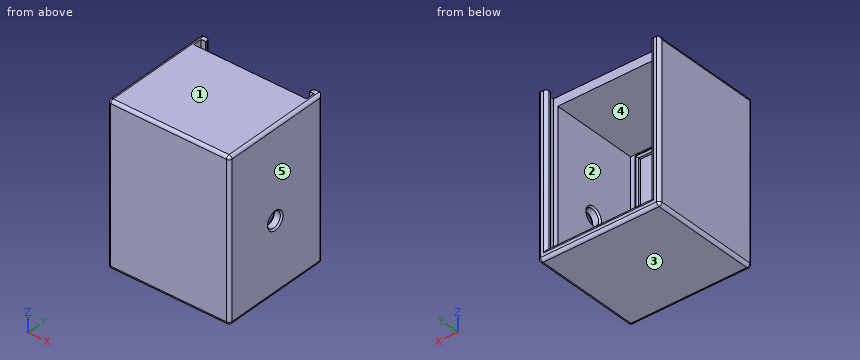
Autodesk Inventor part; units mm, degrees
ref_plane "Work Plane1" through (0, 0, 0) normal (0, 0, 1) x (1, 0, 0)
ref_plane "Work Plane2" through (0, 0, 0) normal (1, 0, 0) x (0, 1, 0)
ref_plane "XZ Plane" through (0, 0, 0) normal (0, 1, 0) x (-1, 0, 0)
sketch "Sketch1" plane through (0, 0, 0) normal (0, 0, 1) x (1, 0, 0)
  line L0 (-41, 37.5) -> (41, 37.5)
  line L1 (41, 37.5) -> (41, -37.5)
  line L2 (41, -37.5) -> (-41, -37.5)
  line L3 (-41, -37.5) -> (-41, 37.5)
  point P0 (0, 0)
  point P1 (0, 37.5)
  point P2 (-41, 0)
  dimension "d0" = 82
  dimension "d1" = 75
extrude "Extrusion1" add sketch "Sketch1" along normal mid plane 107
sketch "Sketch2" plane through (-41, 37.5, 53.5) normal (0, 1, 0) x (1, 0, 0)
  line L0 (0, 107) -> (82, 107)
  line L1 (6, 101) -> (76, 101)
  line L2 (76, 101) -> (76, 6)
  line L3 (76, 6) -> (6, 6)
  line L4 (6, 6) -> (6, 101)
  line L5 (0, 107) -> (0, 0)
  point P0 (41, 53.5)
  point P1 (41, 101)
  point P2 (41, 107)
  point P3 (6, 53.5)
  point P4 (0, 53.5)
  dimension "d4" = 95
  dimension "d5" = 70
extrude "Extrusion2" cut sketch "Sketch2" against normal blind 68
sketch "Sketch3" plane through (0, 0, 53.5) normal (0, 0, 1) x (1, 0, 0)
  line L0 (-35, 37.5) -> (35, 37.5)
  line L1 (35, 37.5) -> (35, 28.5)
  line L2 (35, 28.5) -> (-35, 28.5)
  line L3 (-35, 28.5) -> (-35, 37.5)
  line L4 (41, 37.5) -> (-41, 37.5)
  point P0 (0, 0)
  point P1 (0, 37.5)
  dimension "d14" = 70
  dimension "d15" = 9
extrude "Extrusion3" cut sketch "Sketch3" against normal up to surface (6 mm away)
ref_plane "Work Plane1" through (0, 0, 0) normal (0, 0, 1) x (1, 0, 0)
sketch "Sketch5" plane through (0, 0, 0) normal (0, 0, 1) x (1, 0, 0)
  line L0 (-35, 37.5) -> (-35, -30.5)
  line L1 (-38, 34.5) -> (-35, 34.5)
  line L2 (-35, 34.5) -> (-35, 28.5)
  line L3 (-35, 28.5) -> (-38, 28.5)
  line L4 (-38, 28.5) -> (-38, 34.5)
  point P0 (0, 0)
  dimension "d21" = 3
  dimension "d22" = 6
  dimension "d23" = 3
sketch3d "3D Sketch1"
  line L0 (-35, 37.5, 53.5) -> (-35, 37.5, -47.5)
  line L1 (-35, 37.5, -47.5) -> (35, 37.5, -47.5)
  line L2 (35, 37.5, -47.5) -> (35, 37.5, 53.5)
sweep "Sweep1" cut profiles "Sketch5" path "3D Sketch1"
ref_plane "Work Plane2" through (0, 0, 0) normal (1, 0, 0) x (0, 1, 0)
fillet "Fillet1" radius 2 10 edges at (41, 37.5, 0) (0, 37.5, -53.5) (-41, 37.5, 0) (41, 0, -53.5) (41, 0, 53.5) (-41, 0, 53.5) (-41, 0, -53.5) (35, 37.5, 3) (0, 37.5, -47.5) (-35, 37.5, 3)
fillet "Fillet2" radius 2 8 edges at (40.4142, -37.5, 52.9142) (0, -37.5, 53.5) (-40.4142, -37.5, 52.9142) (-41, -37.5, 0) (-40.4142, -37.5, -52.9142) (0, -37.5, -53.5) (40.4142, -37.5, -52.9142) (41, -37.5, 0)
sketch "Sketch9" plane through (-41, -30.5, 53.5) normal (0, 1, 0) x (1, 0, 0)
  line L0 (10.5, 98.5) -> (71.5, 98.5)
  line L1 (71.5, 98.5) -> (71.5, 8.5)
  line L2 (71.5, 8.5) -> (10.5, 8.5)
  line L3 (10.5, 8.5) -> (10.5, 98.5)
  point P0 (41, 53.5)
  point P1 (41, 96.5)
  point P2 (12.5, 53.5)
  point P3 (10.5, 53.5)
  point P4 (41, 98.5)
  dimension "d48" = 90
  dimension "d49" = 61
extrude "Extrusion5" add sketch "Sketch9" along normal blind 2.5
sketch "Sketch10" plane through (-41, -28, 53.5) normal (0, 1, 0) x (1, 0, 0)
  line L0 (71.5, 98.5) -> (10.5, 98.5)
  line L1 (12.5, 96.5) -> (69.5, 96.5)
  line L2 (69.5, 96.5) -> (69.5, 10.5)
  line L3 (69.5, 10.5) -> (12.5, 10.5)
  line L4 (12.5, 10.5) -> (12.5, 96.5)
  point P0 (41, 53.5)
  point P1 (12.5, 53.5)
  point P2 (41, 96.5)
  dimension "d52" = 57
  dimension "d53" = 86
extrude "Extrusion6" cut sketch "Sketch10" against normal up to surface (2.5 mm away)
fillet "Fillet3" radius 1 8 edges at (0, -28, -45) (0, -28, -43) (-30.5, -28, 0) (-28.5, -28, 0) (0, -28, 43) (0, -28, 45) (28.5, -28, 0) (30.5, -28, 0)
sketch "Sketch12" plane through (35, -30.5, -47.5) normal (-1, 0, 0) x (0, 0, 1)
  circle A0 centre (41, 30) radius 5.25
  line L0 (4.5, 1.5) -> (4.5, 0)
  line L1 (90.5, 0) -> (4.5, 0)
  point P0 (47.5, 30.5)
  dimension "d64" = 36.5
  dimension "d65" = 10.5
  dimension "d66" = 30
extrude "Extrusion7" cut sketch "Sketch12" against normal up to surface (6 mm away)
chamfer "Chamfer1" distance 1 angle 45 1 edges at (41, -0.5, -11.75)
chamfer "Chamfer2" distance 1 angle 45 1 edges at (35, -0.5, -11.75)
Source: CAD feature listing. Evaluate the final solid. Frame: model axes, mm. Face numbers are marked on the shaded views. A direction names the side the tool comes from. Coordinates: 2 decimals unless noted, no trailing zeros. Order: outer loops, then holes, each group sorted by start corner. A loop starts at its lowest first (then second) coordinate and runs counter-clockwise, first axis right, second up. Notation, with made-up numbers: M 45.25,-38 L 82.25,-38 A13 ccw 82.25,-19 Z; hole C 24,-12 d7. An arc over 180 degrees is marked long. Write each question's results on one line, items separated by ' | '. Start each with the question number.
1) Access query for the marked faces 1 and 2. Directions: +Z, -Z, +X, -X, +Y, -Y. A direction counts if a zero-diameter tool reaches every point of the face in a straight line with its end or side. Return the directions, or none.
2) Section query A-A (y = 10). Return the cut outline in (x, z).
3) Line query: line 1 (Y direction, x = 37.4, z = -6.5); line 2 (X direction, y = -13, z = -38); line 3 (Z direction, x = 12, y = 8). Output: solid intervals per line, ascending. Write a range as from..to.
4) Draft query along Z for the marked faces 3, 4 and 5. Return one class per face: released by +Z, released by -Z, zero draft, split by the parting line, or undercut.
5) Section query C-C (y = -0.5). Return the cut outline in (x, z).
6) Contact query for a flat-ended pin moving along its axis: pin 1 Ø6 at (x, z) = (17.5, -39.5) entering from +Y. Output: stop coordinate, or through.
Answers:
1) face 1: +Z, +X, -X, +Y, -Y | face 2: +Y
2) outline: M -41,-51.5 A2 ccw -39,-53.5 L 39,-53.5 A2 ccw 41,-51.5 L 41,51.5 A2 ccw 39,53.5 L -39,53.5 A2 ccw -41,51.5 Z; hole M -35,-47.5 L 35,-47.5 L 35,47.5 L -35,47.5 Z
3) line 1: y = -37.5..-5.75, 4.75..28.5, 34.5..37.5 | line 2: x = -41..-35, 35..41 | line 3: z = -53.5..-47.5, 47.5..53.5
4) face 3: released by -Z | face 4: undercut | face 5: zero draft
5) outline: M -41,-51.5 A2 ccw -39,-53.5 L 39,-53.5 A2 ccw 41,-51.5 L 41,-12.75 L 40,-11.75 L 36,-11.75 L 35,-12.75 L 35,-47.5 L -35,-47.5 L -35,47.5 L 35,47.5 L 35,-0.25 L 36,-1.25 L 40,-1.25 L 41,-0.25 L 41,51.5 A2 ccw 39,53.5 L -39,53.5 A2 ccw -41,51.5 Z
6) pin 1: stops at y = -30.5
